The listing builds one solid part. Answer for the finished solid, in the listing's coordinates (mm). A direction names the side the tool comes from. Round coordinates to 2 decimals unless told otherwise and drop trailing zeros.
from build123d import *
from build123d.topology import SkipClean

# Parameters (mm, degrees)
SKETCH_1_W          = 10
SKETCH_1_H          = 2
REVOLVE_1_ANGLE     = 180
SKETCH_2_R          = 3
EXTRUDE_1_DEPTH     = 3
SKETCH_3_R          = 2
EXTRUDE_2_DEPTH     = 8
SKETCH_4_R          = 2
EXTRUDE_3_DEPTH     = 8
HOLE_WIZARD_1_D     = 2
HOLE_WIZARD_1_DEPTH = 8
RIB_START           = 3
RIB_1_DEPTH         = 8
SKETCH_8_R          = 1
CUT_EXTRUDE_1_DEPTH = 10
CUT_EXTRUDE_START   = -11
SKETCH_9_R          = 1
CUT_EXTRUDE_2_DEPTH = 11
SKETCH_10_W         = 2
SKETCH_10_H         = 9.392270145
SKETCH_11_W         = 2
SKETCH_11_H         = 9.392270145
CUT_REVOLVE_2_ANGLE = 112
CUT_EXTRUDE_4_DEPTH = 10


# Read off the part's stored shape, not the designer's step: 筋1
with BuildPart() as part:
    # 草图1 → 旋转1 (revolve)
    with BuildSketch(Plane(origin=(0, 0, 0), x_dir=(0, -1, 0), z_dir=(-0.422618261740697, 0, 0.9063077870366512))):
        with Locations((-8, 22)):
            Rectangle(SKETCH_1_W, SKETCH_1_H)
    revolve(axis=Axis((0, 13, 0), (0, 1, 0)), revolution_arc=REVOLVE_1_ANGLE)

    # 草图2 → 凸台-拉伸1 (add)
    with BuildSketch(Plane.XZ.offset(-3)):
        with BuildLine():
            Line((-7.687738047, 3.187259937), (-15.625582333, 9.847902149))
            ThreePointArc((-15.625582333, 9.847902149), (-15.933724417, 13.369982281), (-12.411644285, 13.678124365))
            Line((-12.411644285, 13.678124365), (-4.14278761, 6.739729779))
            ThreePointArc((-4.14278761, 6.739729779), (-3.077381738, 6.599466435), (-2.5, 7.505774222))
            Line((-2.5, 7.505774222), (-2.5, 18.3))
            ThreePointArc((-2.5, 18.3), (0, 20.8), (2.5, 18.3))
            Line((2.5, 18.3), (2.5, 16.292228073))
            ThreePointArc((2.5, 16.292228073), (2.740367594, 15.341599967), (3.403693795, 14.619472052))
            Line((3.403693795, 14.619472052), (10.364457725, 10.057462653))
            Line((10.364457725, 10.057462653), (14.091579804, 7.614747152))
            ThreePointArc((14.091579804, 7.614747152), (15.044154935, 7.292674514), (16.033062771, 7.474859732))
            Line((16.033062771, 7.474859732), (20.071872558, 9.358025555))
            Line((20.071872558, 9.358025555), (20.845720003, 9.718845484))
            ThreePointArc((20.845720003, 9.718845484), (9.719853203, -20.84608682), (-20.845079102, -9.72022002))
            Line((-20.845079102, -9.72022002), (-8.687048035, -4.051325027))
            ThreePointArc((-8.687048035, -4.051325027), (-7.926279341, -3.430713127), (-7.552514649, -2.522843041))
            Line((-7.552514649, -2.522843041), (-6.993603119, 1.371009596))
            ThreePointArc((-6.993603119, 1.371009596), (-7.105101968, 2.369164428), (-7.687738047, 3.187259937))
        make_face()
        with Locations(Location((0.000320451, -0.000687268, 0), (0, 0, 90))):
            Circle(SKETCH_2_R, mode=Mode.SUBTRACT)
    extrude(amount=EXTRUDE_1_DEPTH)

    # 草图3 → 凸台-拉伸2 (add)
    with BuildSketch(Plane(origin=(0, 3, 0), x_dir=(-1, 0, 0), z_dir=(0, 1, 0))):
        with Locations(Location((14.018613309, 11.763013257, 0), (0, 0, 90))):
            Circle(SKETCH_3_R)
    extrude(amount=EXTRUDE_2_DEPTH)

    # 草图4 → 凸台-拉伸3 (add)
    with BuildSketch(Plane(origin=(0, 3, 0), x_dir=(-1, 0, 0), z_dir=(0, 1, 0))):
        with Locations(Location((0, 18.3, 0), (0, 0, 90))):
            Circle(SKETCH_4_R)
    extrude(amount=EXTRUDE_3_DEPTH)

    # 孔1
    with Locations(Plane(origin=(0, 11, 0), x_dir=(1, 0, 0), z_dir=(0, 1, 0))):
        with Locations((0, -18.3), (-14.018613309, -11.763013257)):
            Hole(HOLE_WIZARD_1_D / 2, depth=HOLE_WIZARD_1_DEPTH)

    # 筋1 outline → 筋1 (add)
    with BuildSketch(Plane(origin=(0, 0, 0), x_dir=(1, 0, 0), z_dir=(0, 1, 0)).offset(RIB_START)):
        with BuildLine():
            ThreePointArc((12.553349452, 16.834886918), (8.874983497, 19.032463528), (4.827134087, 20.437680312))
            Line((4.827134087, 20.437680312), (4.827134087, 19.816628788))
            Line((4.827134087, 19.816628788), (12.077596383, 16.435682694))
            Line((12.077596383, 16.435682694), (12.553349452, 16.834886918))
        make_face()
    extrude(amount=RIB_1_DEPTH)

    # 草图8 → 切除-拉伸1 (cut)
    with BuildSketch(Plane.XZ):
        with Locations(Location((-14.018613309, 11.763013257, 0), (0, 0, 90))):
            Circle(SKETCH_8_R)
    extrude(amount=-CUT_EXTRUDE_1_DEPTH, mode=Mode.SUBTRACT)

    # 草图9 → 切除-拉伸2 (cut)
    with BuildSketch(Plane(origin=(0, 11, 0), x_dir=(1, 0, 0), z_dir=(0, 1, 0)).offset(CUT_EXTRUDE_START)):
        with Locations(Location((0, -18.3, 0), (0, 0, 270))):
            Circle(SKETCH_9_R)
    extrude(amount=CUT_EXTRUDE_2_DEPTH, mode=Mode.SUBTRACT)

    # 草图10 → 旋转15 (revolve)
    with SkipClean():  # the faces are left unmerged after this step: merging them gives an invalid solid
        with BuildSketch(Plane(origin=(0, 0, 0), x_dir=(0.9063077870366516, 0, 0.4226182617406962), z_dir=(-0.4226182617406962, 0, 0.9063077870366516)), mode=Mode.PRIVATE) as revolve_15_sk:
            with Locations((-22, 4.696135073)):
                Rectangle(SKETCH_10_W, SKETCH_10_H)
        revolve(revolve_15_sk.sketch.rotate(Axis((0, 0, 0), (0, 1, 0)), 281.710962798), axis=Axis((0, 0, 0), (0, 1, 0)))

    # 草图11 → 切除-旋转2 (revolve, cut)
    with BuildSketch(Plane(origin=(0, 0, 0), x_dir=(0.9063077870366513, 0, 0.42261826174069694), z_dir=(-0.42261826174069694, 0, 0.9063077870366513))):
        with Locations((22, 4.696135073)):
            Rectangle(SKETCH_11_W, SKETCH_11_H)
    revolve(axis=Axis((0, 0, 0), (0, -1, 0)), revolution_arc=CUT_REVOLVE_2_ANGLE, mode=Mode.SUBTRACT)

    # 草图12 → 切除-拉伸4 (cut)
    with BuildSketch(Plane.XZ):
        Polygon((9.548814336, 2.649444135), (1.884926874, -10.672654147), (11.982316999, -16.481443418), (19.646204461, -3.159345136), align=None)
    extrude(amount=-CUT_EXTRUDE_4_DEPTH, mode=Mode.SUBTRACT)


solid = part.part
1. Straight lines are drawn through the part: line 1 along X through (y, z) = (9.25, -16.5); line 2 along X through (y, z) = (6.5, 18.3); line 3 along X through (y, z) = (2.25, 2). For each, find the intervals that lie inside material, in ascending order.
Geometry says:
line 1: x = -16.02 to -12.99, 11.94 to 12.15, 12.99 to 16.02
line 2: x = -2 to -1, 1 to 2
line 3: x = -22.91 to -20.9, -7 to -2.24, 2.24 to 9.18, 10.68 to 22.91
2. Section C-C on y = 7 is taken. Give the number of separate pieces and of enclosed holes in the cut face, plus the area to 3 significant figures.
Geometry says:
separate pieces: 3
enclosed holes: 2
area: 216 mm2
3. For a pull along Z with two mould halves and no side action, classify faces 5 (the face through (-0.383, 5.423, 19.224)), 6 (the face through (-3.092, 1.521, 6.593)), 7 (the face through (-13.932, 1.521, -6.497)), 8 (the face through (8.7, 11, -18.6)) as released by +Z, released by -Z, zero draft, split by the parting line, or undercut.
Geometry says:
face 5: undercut
face 6: released by +Z
face 7: undercut
face 8: zero draft
4. A tool of negligible diameter and unlimited length cuts with its end or side. For faces 1 (the face through (-8.34, 1.52, 10.26)), 2 (the face through (-7.935, 1.521, -3.442)), 3 (the face through (-21, 9.392, 3)), 4 (the face through (1, 3, -4)), from which of +Z, -Z, +X, -X, +Y, -Y can it reach the whole face along a straight path? Write none if from no direction.
Geometry says:
face 1: +Z, +Y, -Y
face 2: +Y, -Y
face 3: +Z, -X, +Y
face 4: +Y
5. Given pin 1 (2 mm diameter, centred on y = 6, z = 13.5, fed in from -X); pin 2 (1.6 mm diameter, centred on y = 1, z = 17.5, fed in from +X); pin 3 (3 mm diameter, centred on x = 1, z = 19, fed in from +Y), each flat-ended and moving along its own axis, determine where each tip first touches the part or whether it passes through.
Geometry says:
pin 1: stops at x = -19.31
pin 2: stops at x = 2.5
pin 3: stops at y = 11
